Design review of the part built by this model. Coordinates are the model's own, in mm. Face numbers are marked on the shaded views. A direction names the side the tool comes from. Give positions to 0.01 mm unless a question says otherwise; leave off trailing zeros. Order: outer loops, then holes, each group sorted by start corner. A loop starts at its lowest first (then second) coordinate and runs counter-clockwise, first axis right, second up.
```python
from build123d import *

# Parameters (mm, degrees)
EXTRU_MINCE1_DEPTH      = 6
EXTRU_MINCE2_DEPTH      = 7.5
CONG_1_R                = 4
CONG_2_R                = 1
ESQUISSE3_R             = 1.5
ENL_V_MAT_EXTRU_1_DEPTH = 57.387055252


with BuildPart() as part:
    # Esquisse1 → Extru.-Mince1 (new, symmetric)
    with BuildSketch(Plane.XY):
        with BuildLine():
            Line((0, -45), (0, -34))
            Line((0, -34), (-13, -34))
            ThreePointArc((-13, -34), (-15.828427125, -32.828427125), (-17, -30))
            Line((-17, -30), (-17, 30))
            ThreePointArc((-17, 30), (-15.828427125, 32.828427125), (-13, 34))
            Line((-13, 34), (0, 34))
            Line((0, 34), (0, 45))
            Line((0, 45), (-1.5, 45))
            Line((-1.5, 45), (-1.5, 35.5))
            Line((-1.5, 35.5), (-13, 35.5))
            ThreePointArc((-13, 35.5), (-16.889087297, 33.889087297), (-18.5, 30))
            Line((-18.5, 30), (-18.5, -30))
            ThreePointArc((-18.5, -30), (-16.889087297, -33.889087297), (-13, -35.5))
            Line((-13, -35.5), (-1.5, -35.5))
            Line((-1.5, -35.5), (-1.5, -45))
            Line((-1.5, -45), (0, -45))
        make_face()
    extrude(amount=EXTRU_MINCE1_DEPTH, both=True)

    # Esquisse2 → Extru.-Mince2 (add, symmetric)
    with BuildSketch(Plane(origin=(0, 0, 0), x_dir=(1, 0, 0), z_dir=(0, 1, 0))):
        with BuildLine():
            Line((-17, -6), (-17, -23))
            ThreePointArc((-17, -23), (-15.828427125, -25.828427125), (-13, -27))
            Line((-13, -27), (-2, -27))
            Line((-2, -27), (-2, -28.5))
            Line((-2, -28.5), (-13, -28.5))
            ThreePointArc((-13, -28.5), (-16.889087297, -26.889087297), (-18.5, -23))
            Line((-18.5, -23), (-18.5, -6))
            Line((-18.5, -6), (-17, -6))
        make_face()
    extrude(amount=EXTRU_MINCE2_DEPTH, both=True)

    # Congé1
    cong_1_edges = [part.edges().sort_by_distance(p)[0] for p in [
        (-0.75, 45, -6),
        (-0.75, 45, 6),
        (-2, 7.5, 27.75),
        (-2, -7.5, 27.75),
        (-0.75, -45, -6),
        (-0.75, -45, 6),
        (-17.75, -7.5, 6),
        (-17.75, 7.5, 6),
    ]]
    fillet(cong_1_edges, radius=CONG_1_R)

    # Congé2
    cong_2_edges = [part.edges().sort_by_distance(p)[0] for p in [
        (-1.5, -35.5, 0),
        (-1.5, 35.5, 0),
    ]]
    fillet(cong_2_edges, radius=CONG_2_R)

    # Esquisse3 → Enlèv. mat.-Extru.1 (cut, through all)
    with BuildSketch(Plane(origin=(0, 0, 0), x_dir=(0, 0, -1), z_dir=(1, 0, 0))):
        with Locations(Location((0, 40, 0), (0, 0, 90))):
            Circle(ESQUISSE3_R)
        with Locations(Location((0, -40, 0), (0, 0, 90))):
            Circle(ESQUISSE3_R)
    extrude(amount=-ENL_V_MAT_EXTRU_1_DEPTH, mode=Mode.SUBTRACT)


solid = part.part
```
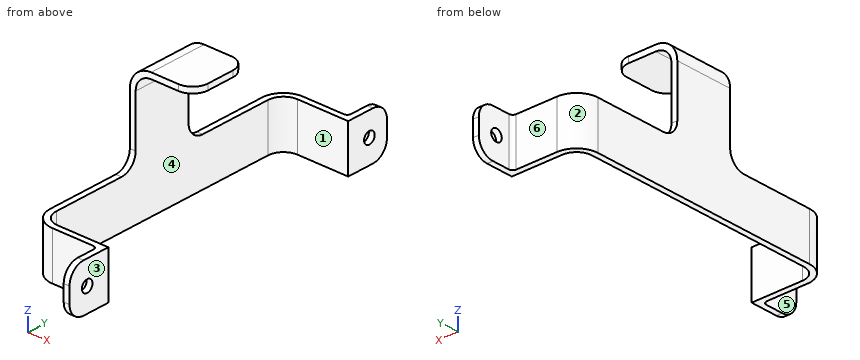
1. Take a section at B-B (y = -40). State the section outline as (x, z) points.
Recorded:
outline: (-1.5, -6) - (0, -6) - (0, -1.5) - (-1.5, -1.5) - close; (-1.5, 1.5) - (0, 1.5) - (0, 6) - (-1.5, 6) - close
2. For pin 1 (10 mm diameter, centred on y = 12, z = 10, fed in from +X); pin 2 (8.5 mm diameter, centred on x = -6, z = -1, fed in from +Y); pin 3 (4 mm diameter, centred on y = -42.5, z = 0.5, fed in from -X), all flat-tipped, find the tip position at first contact; note any pin that passes through.
Recorded:
pin 1: stops at x = -17
pin 2: stops at y = 35.84
pin 3: stops at x = -1.5
3. Draft analysis for pull direction Y (two halves, no side actions). For the marked faces 1, 2 and 3, state which applies: pulls with the +Y half, pulls with the -Y half, needs draft (parallel to the pull), parting line crosses it, or undercut.
Recorded:
face 1: undercut
face 2: pulls with the +Y half
face 3: needs draft
4. Take a section at C-C (z = 0). State the section outline as (x, y) points.
Recorded:
outline: (-18.5, -30) arc R5.5 ccw to (-13, -35.5) - (-2.5, -35.5) arc R1 cw to (-1.5, -36.5) - (-1.5, -38.5) - (0, -38.5) - (0, -34) - (-13, -34) arc R4 cw to (-17, -30) - (-17, 30) arc R4 cw to (-13, 34) - (0, 34) - (0, 38.5) - (-1.5, 38.5) - (-1.5, 36.5) arc R1 cw to (-2.5, 35.5) - (-13, 35.5) arc R5.5 ccw to (-18.5, 30) - close; (-1.5, -45) - (0, -45) - (0, -41.5) - (-1.5, -41.5) - close; (-1.5, 41.5) - (0, 41.5) - (0, 45) - (-1.5, 45) - close
5. Machinability: for the marked faces 4, 5 and 6, which of the approach directions +Z, -Z, +X, -X, +Y, -Y give a long, thin tool a straight path to every point of the face, cutting with its end or side? Answer none if there is none.
Recorded:
face 4: -Z, +X
face 5: +Z, -Z, -X, -Y
face 6: +Z, -Z, -X, +Y
6. Take a section at D-D (y = 23). State the section outline as (x, z) points.
Recorded:
outline: (-18.5, -6) - (-17, -6) - (-17, 6) - (-18.5, 6) - close
7. For line 1 along Y through (x, z) = (-3.5, -3.5); line 2 along Z through (x, y) = (-0.5, -40); line 3 along X through (y, z) = (-29.5, 4.5), list the stretches that pass through material, from the lowest coordinate up.
Recorded:
line 1: y = -35.5 to -34, 34 to 35.5
line 2: z = -6 to -1.5, 1.5 to 6
line 3: x = -18.5 to -17
8. Take a section at A-A (x = -10.25). State the section outline as (y, z) points.
Recorded:
outline: (-35.5, -6) - (-34, -6) - (-34, 6) - (-35.5, 6) - close; (-7.5, 27) - (7.5, 27) - (7.5, 28.5) - (-7.5, 28.5) - close; (34, -6) - (35.5, -6) - (35.5, 6) - (34, 6) - close
